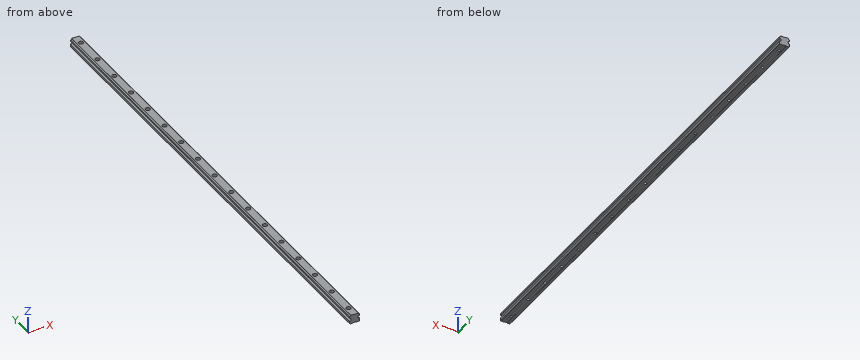
from build123d import *

# Parameters (mm, degrees)
RESSALTO_EXTRUS_O1_DEPTH = 1000
ESBO_O2_R                = 2.87
CORTE_EXTRUS_O1_DEPTH    = 17.57
ESBO_O3_R                = 4.715
CORTE_EXTRUS_O2_DEPTH    = 8.49


with BuildPart() as part:
    # Esboço1 → Ressalto-extrusão1 (new body)
    with BuildSketch(Plane(origin=(0, 0, 0), x_dir=(1, 0, 0), z_dir=(0, 1, 0))):
        with BuildLine():
            Line((-10.048, -3.265), (-10.048, -6.485))
            Line((-10.048, -6.485), (-9.645814792, -6.485))
            ThreePointArc((-9.645814792, -6.485), (-8.23160123, -7.070786438), (-7.645814792, -8.485))
            Line((-7.645814792, -8.485), (-7.645814792, -8.985))
            Line((-7.645814792, -8.985), (7.652, -8.985))
            Line((7.652, -8.985), (7.652, -8.485))
            ThreePointArc((7.652, -8.485), (8.237786438, -7.070786438), (9.652, -6.485))
            Line((9.652, -6.485), (10.152, -6.485))
            Line((10.152, -6.485), (10.152, -3.265))
            ThreePointArc((10.152, -3.265), (7.052, -0.165), (10.152, 2.935))
            Line((10.152, 2.935), (10.152, 8.315))
            Line((10.152, 8.315), (9.152, 9.315))
            Line((9.152, 9.315), (3.667, 9.315))
            Line((3.667, 9.315), (3.667, 8.585))
            Line((3.667, 8.585), (-3.563, 8.585))
            Line((-3.563, 8.585), (-3.563, 9.315))
            Line((-3.563, 9.315), (-9.048, 9.315))
            Line((-9.048, 9.315), (-10.048, 8.315))
            Line((-10.048, 8.315), (-10.048, 2.935))
            ThreePointArc((-10.048, 2.935), (-6.948, -0.165), (-10.048, -3.265))
        make_face()
    extrude(amount=-RESSALTO_EXTRUS_O1_DEPTH)

    # Esboço2 → Corte-extrusão1 (cut)
    with BuildSketch(Plane(origin=(0, 0, -8.585), x_dir=(-1, 0, 0), z_dir=(0, 0, -1))):
        with Locations((0, -19.745)):
            Circle(ESBO_O2_R)
        with Locations((0, -79.655)):
            Circle(ESBO_O2_R)
        with Locations((0, -139.565)):
            Circle(ESBO_O2_R)
        with Locations((0, -199.475)):
            Circle(ESBO_O2_R)
        with Locations((0, -259.385)):
            Circle(ESBO_O2_R)
        with Locations((0, -319.295)):
            Circle(ESBO_O2_R)
        with Locations((0, -379.205)):
            Circle(ESBO_O2_R)
        with Locations((0, -439.115)):
            Circle(ESBO_O2_R)
        with Locations((0, -499.025)):
            Circle(ESBO_O2_R)
        with Locations((0, -558.935)):
            Circle(ESBO_O2_R)
        with Locations((0, -618.845)):
            Circle(ESBO_O2_R)
        with Locations((0, -678.755)):
            Circle(ESBO_O2_R)
        with Locations((0, -738.665)):
            Circle(ESBO_O2_R)
        with Locations((0, -798.575)):
            Circle(ESBO_O2_R)
        with Locations((0, -858.485)):
            Circle(ESBO_O2_R)
        with Locations((0, -918.395)):
            Circle(ESBO_O2_R)
        with Locations((0, -978.305)):
            Circle(ESBO_O2_R)
    extrude(amount=-CORTE_EXTRUS_O1_DEPTH, mode=Mode.SUBTRACT)

    # Esboço3 → Corte-extrusão2 (cut)
    with BuildSketch(Plane.XY.offset(8.985)):
        with Locations((0.003092604, -19.745)):
            Circle(ESBO_O3_R)
        with Locations((0.003092604, -79.645)):
            Circle(ESBO_O3_R)
        with Locations((0.003092604, -139.545)):
            Circle(ESBO_O3_R)
        with Locations((0.003092604, -199.445)):
            Circle(ESBO_O3_R)
        with Locations((0.003092604, -259.345)):
            Circle(ESBO_O3_R)
        with Locations((0.003092604, -319.245)):
            Circle(ESBO_O3_R)
        with Locations((0.003092604, -379.145)):
            Circle(ESBO_O3_R)
        with Locations((0.003092604, -439.045)):
            Circle(ESBO_O3_R)
        with Locations((0.003092604, -498.945)):
            Circle(ESBO_O3_R)
        with Locations((0.003092604, -558.845)):
            Circle(ESBO_O3_R)
        with Locations((0.003092604, -618.745)):
            Circle(ESBO_O3_R)
        with Locations((0.003092604, -678.645)):
            Circle(ESBO_O3_R)
        with Locations((0.003092604, -738.545)):
            Circle(ESBO_O3_R)
        with Locations((0.003092604, -798.445)):
            Circle(ESBO_O3_R)
        with Locations((0.003092604, -858.345)):
            Circle(ESBO_O3_R)
        with Locations((0.003092604, -918.245)):
            Circle(ESBO_O3_R)
        with Locations((0.003092604, -978.145)):
            Circle(ESBO_O3_R)
    extrude(amount=-CORTE_EXTRUS_O2_DEPTH, mode=Mode.SUBTRACT)


solid = part.part
Input: part model. Units: mm. Frame: model coordinates. Give positions to 0.01 mm unless a question says otherwise; leave off trailing zeros. Write each loop counter-clockwise with the first axis right and the second up, starting at its lowest first coordinate (ties: lowest second). Pieces come first, ordered by that corner, then holes. Notation, with made-up numbers: M 53,4.25 L 66,4.25 A23 ccw 66,18.25 Z; hole C 30,83.25 d7. An arc over 180 degrees is marked long. Use one line per item in the form item = value.
1. Cut plane A-A on y = -225.5. Return loops of the section in (x, z) (3 decimals), and give its area (3 significant figures).
Outcome:
outline = M -10.048,-8.315 L -9.048,-9.315 L -3.563,-9.315 L -3.563,-8.585 L 3.667,-8.585 L 3.667,-9.315 L 9.152,-9.315 L 10.152,-8.315 L 10.152,-2.935 A3.1 cw 10.152,3.265 L 10.152,6.485 L 9.652,6.485 A2 cw 7.652,8.485 L 7.652,8.985 L -7.646,8.985 L -7.646,8.485 A2 cw -9.646,6.485 L -10.048,6.485 L -10.048,3.265 A3.1 cw -10.048,-2.935 Z
area = 323 mm²
2. First-contact query: P1, Ø7.5, axis at x = -1.5, y = -197.5, coming from the +Z side (3 decimals); P2, Ø4, axis at x = -1, y = -180, coming from the -Z side (3 decimals); P3, Ø4, axis at y = -147, z = 1, coming from the +X side; P4, Ø7.5, axis at x = 0, y = -738.54, coming from the +Z side (3 decimals). Flat tips, straight axial feed; report the tip coordinate or a pass-through.
Outcome:
P1 = 8.985
P2 = -8.585
P3 = 8.9
P4 = 0.495
3. Ray query, L1, parallel to X at y = -79.5, z = -0.5; L2, parallel to X at y = -416, z = -0.5; L3, parallel to X at y = -90, z = 2. Return the intervals inside material, ascending.
Outcome:
L1 = -7.02 to -2.87, 2.87 to 7.12
L2 = -7.02 to 7.12
L3 = -7.55 to 7.65
